Verification items for the finished model (mm, model axes). Round coordinates to 2 decimals unless told otherwise and drop trailing zeros. Loops run counter-clockwise (first coordinate to the right, second up) from the corner with the lowest first, then second, coordinate; pieces in that order, holes last. Notation, with made-up numbers: (-27, 5) - (29, 5) arc R11 ccw to (29, 18) - close; hole circle Ø8 at (-1.75, -18.75). An arc over 180 degrees is marked (long way). Use CSV: the item, a comma, the result in double quotes.
```python
from build123d import *

# Parameters (mm, degrees)
F0_W     = 52.7011975646
F0_H     = 151.7794504762
F2_R     = 5.08
F3_W     = 15.9061774611
F3_H     = 6.3241422176
F3_W_2   = 16.6727416217
F3_H_2   = 6.5157860518
F3_W_3   = 15.9061811864
F4_DEPTH = 58.42


with BuildPart() as f1:
    # F0 (on Front) → F1 (revolve)
    with BuildSketch(Plane.XZ):
        with Locations((-26.3505987823, -0.0958181918)):
            Rectangle(F0_W, F0_H)
    revolve(axis=Axis((-52.7011975646, 0, -0.0958181918), (0, 0, 1)))

    # F2
    f2_edges = [f1.edges().sort_by_distance(p)[0] for p in [
        (-105.402395, 0, 75.793907),
        (-105.402395, 0, -75.985543),
    ]]
    fillet(f2_edges, radius=F2_R)

    # F3 (on Front) → F4 (join)
    with BuildSketch(Plane.XZ):
        with Locations((-76.2136913836, -67.6491707563)):
            Rectangle(F3_W, F3_H)
        with Locations((-56.4746949822, -67.7449926734)):
            Rectangle(F3_W_2, F3_H_2)
        with Locations((-36.3524202257, -67.7449926734)):
            Rectangle(F3_W_3, F3_H_2)
    extrude(amount=F4_DEPTH)


solid = f1.part
```
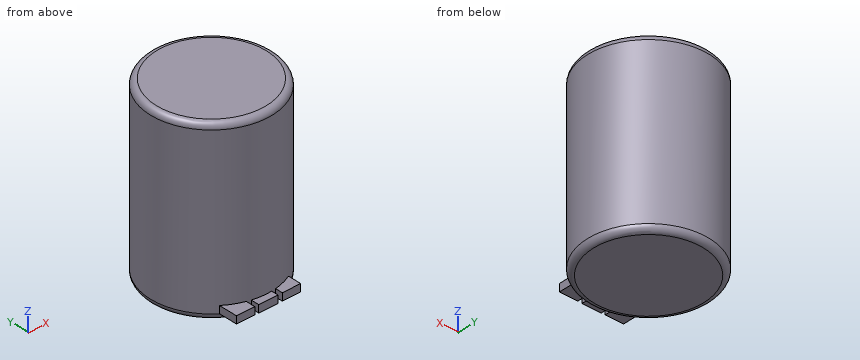
1) Thickness scan on probe 1 along Z at (x, y) = (-13, 27); probe 2 along X at (y, z) = (4.5, 47.5); probe 3 along Y at (x, z) = (-20.5, 59). Record the ranges inside material, lowest first. Write a range as [from, to].
Returned:
probe 1,"z = [-75.97, 75.78]"
probe 2,"x = [-105.21, -0.19]"
probe 3,"y = [-41.72, 41.72]"
2) Gauge pin test, flat ends, axial feed: pin 1 Ø1 at (x, z) = (-64.5, 23) entering from +Y; pin 2 Ø10 at (y, z) = (34, 1.5) entering from -X; pin 3 Ø10 at (x, z) = (-43.5, -27) entering from -Y. Record the tip position at first contact, or that the pin passes through.
Returned:
pin 1,"stops at y = 51.48"
pin 2,"stops at x = -96.71"
pin 3,"stops at y = -52.53"
3) Cross-section at A-A, the plane z = -52. Record the cut outline in (x, y).
Returned:
outline,"circle Ø105.4 at (-52.7, 0)"
